```python
from build123d import *

# Parameters (mm, degrees)
SKETCH1_R           = 1.9
SKETCH1_R_2         = 1.500800978
SKETCH1_R_3         = 1.5
BOSS_EXTRUDE1_DEPTH = 5


with BuildPart() as part:
    # Sketch1 → Boss-Extrude1 (new body)
    with BuildSketch(Plane.XY):
        with BuildLine():
            Line((-6.997330295, -256.787047369), (-14.00854399, -256.787047369))
            ThreePointArc((-14.00854399, -256.787047369), (-15.422757553, -256.201260932), (-16.00854399, -254.787047369))
            Line((-16.00854399, -254.787047369), (-16.00854399, -227.870547218))
            ThreePointArc((-16.00854399, -227.870547218), (-15.422757553, -226.456333656), (-14.00854399, -225.870547218))
            Line((-14.00854399, -225.870547218), (-6.997330295, -225.870547218))
            ThreePointArc((-6.997330295, -225.870547218), (-5.583116733, -225.284760781), (-4.997330295, -223.870547218))
            Line((-4.997330295, -223.870547218), (-4.997330295, -217.870547218))
            ThreePointArc((-4.997330295, -217.870547218), (-4.411543858, -216.456333656), (-2.997330295, -215.870547218))
            Line((-2.997330295, -215.870547218), (3.002669705, -215.870547218))
            ThreePointArc((3.002669705, -215.870547218), (4.416883267, -216.456333656), (5.002669705, -217.870547218))
            Line((5.002669705, -217.870547218), (5.002669705, -223.870547218))
            ThreePointArc((5.002669705, -223.870547218), (5.588456142, -225.284760781), (7.002669705, -225.870547218))
            Line((7.002669705, -225.870547218), (7.505072862, -225.870547218))
            ThreePointArc((7.505072862, -225.870547218), (8.919286424, -226.456333656), (9.505072862, -227.870547218))
            Line((9.505072862, -227.870547218), (9.505072862, -254.787047369))
            ThreePointArc((9.505072862, -254.787047369), (8.919286424, -256.201260932), (7.505072862, -256.787047369))
            Line((7.505072862, -256.787047369), (7.002669705, -256.787047369))
            ThreePointArc((7.002669705, -256.787047369), (5.588456142, -257.372833807), (5.002669705, -258.787047369))
            Line((5.002669705, -258.787047369), (5.002669705, -264.787047369))
            ThreePointArc((5.002669705, -264.787047369), (4.416883267, -266.201260932), (3.002669705, -266.787047369))
            Line((3.002669705, -266.787047369), (-2.997330295, -266.787047369))
            ThreePointArc((-2.997330295, -266.787047369), (-4.411543858, -266.201260932), (-4.997330295, -264.787047369))
            Line((-4.997330295, -264.787047369), (-4.997330295, -258.787047369))
            ThreePointArc((-4.997330295, -258.787047369), (-5.583116733, -257.372833807), (-6.997330295, -256.787047369))
        make_face()
        with Locations((0, -261.876090751)):
            Circle(SKETCH1_R, mode=Mode.SUBTRACT)
        with Locations((5.002669705, -234.375086095)):
            Circle(SKETCH1_R_2, mode=Mode.SUBTRACT)
        with Locations((-10.805767266, -234.375086095)):
            Circle(SKETCH1_R_2, mode=Mode.SUBTRACT)
        with Locations(Location((0, -220.781503837, 0), (0, 0, 180))):
            Circle(SKETCH1_R, mode=Mode.SUBTRACT)
        with Locations((5.002669705, -248.275086095)):
            Circle(SKETCH1_R_3, mode=Mode.SUBTRACT)
        with Locations((-10.797330295, -248.275086095)):
            Circle(SKETCH1_R_3, mode=Mode.SUBTRACT)
    extrude(amount=BOSS_EXTRUDE1_DEPTH)


solid = part.part
```
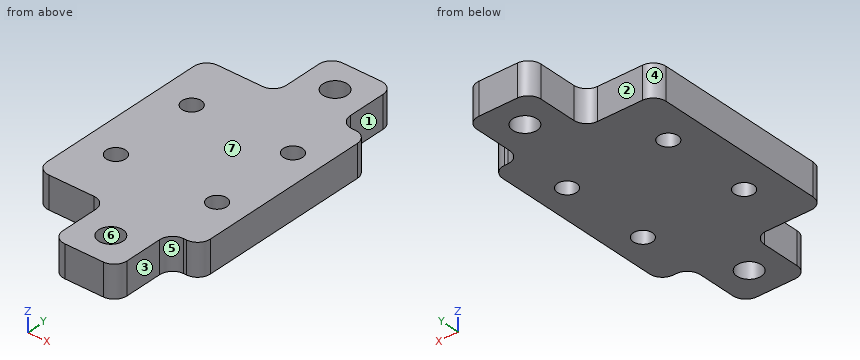
The model under review builds one solid part; all positions refer to its coordinate system, in mm. Face numbers are marked on the shaded views. A direction names the side the tool comes from. Coordinates: 2 decimals unless noted, no trailing zeros. Write each loop counter-clockwise with the first axis right and the second up, starting at its lowest first coordinate (ties: lowest second). Pieces come first, ordered by that corner, then holes. Notation, with made-up numbers: (36, 36.5) - (93, 36.5) arc R31 cw to (93, 66.5) - close; hole circle Ø7 at (15, -5). An arc over 180 degrees is marked (long way). Write item = value, one per line.
(1) Consider section B-B, the plane z = 2.65. State how many separate pieces and enclosed holes the cut face has, then the cut area to 3 significant figures.
Result sheet:
separate_pieces = 1
enclosed_holes = 6
area = 934 mm^2
(2) For line 1 (X direction, y = -234.5, z = 1.75); line 2 (Y direction, x = 4.5, z = 4.35); line 3 (X direction, y = -218, z = 4.1), list the stretches that pass through material, from the lowest coordinate up. Write a range as [from, to].
Result sheet:
line_1 = [-16.01, -12.3], [-9.31, 3.51], [6.5, 9.51]
line_2 = [-266.11, -249.69], [-246.86, -235.79], [-232.96, -216.54]
line_3 = [-5, 5]
(3) Machinability: for the marked faces 1, 2 and 3, which of the approach directions +Z, -Z, +X, -X, +Y, -Y give a long, thin tool a straight path to every point of the face, cutting with its end or side? Answer none if there is none.
Result sheet:
face_1 = +Z, -Z, +X, +Y
face_2 = +Z, -Z, -X, +Y
face_3 = +Z, -Z, +X, -Y
(4) For P1, Ø2.5, axis at x = -10.81, y = -234.38, coming from the -Z side; P2, Ø0.6, axis at x = 7, z = 3.5, coming from the -Y side; P3, Ø2.5, axis at y = -222, z = 3.5, coming from the -X side; P4, Ø2.5, axis at x = -10, z = 3.5, coming from the +Y side, all flat-tipped, find the tip position at first contact; note any pin that passes through.
Result sheet:
P1 = through
P2 = -256.81
P3 = -5
P4 = -225.87
(5) Consider section C-C, the plane x = -6.5. Give the boundary of the cut face in (y, z).
Result sheet:
outline = (-256.85, 0) - (-225.81, 0) - (-225.81, 5) - (-256.85, 5) - close
(6) Consider section A-A, the plane x = 0. Give the boundary of the cut face in (y, z), then the cut area to 3 significant figures.
Result sheet:
outline = (-266.79, 0) - (-263.78, 0) - (-263.78, 5) - (-266.79, 5) - close; (-259.98, 0) - (-222.68, 0) - (-222.68, 5) - (-259.98, 5) - close; (-218.88, 0) - (-215.87, 0) - (-215.87, 5) - (-218.88, 5) - close
area = 217 mm^2
(7) Mouldability with a two-part tool opening along Y and no side actions: class the marked faces 4, 5, 6 and 7 as pulls with the +Y half, pulls with the -Y half, needs draft (parallel to the pull), parting line crosses it, or undercut.
Result sheet:
face_4 = pulls with the +Y half
face_5 = pulls with the -Y half
face_6 = undercut
face_7 = needs draft
